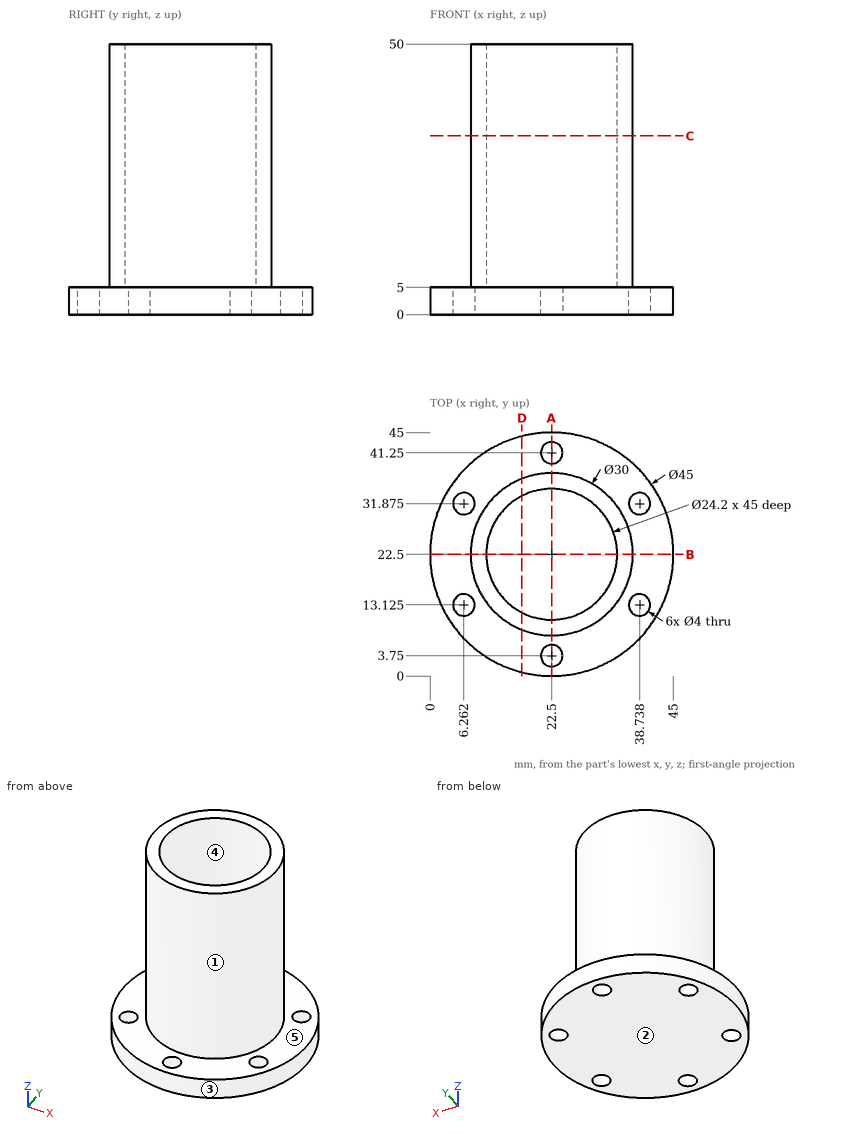
Design review of the part shown in the three views and the two pictorial views. Dimensions are in mm from the part's minimum x, y and z. A direction names the side the tool comes from. Round coordinates to 2 decimals unless told otherwise and drop trailing zeros. Write each loop counter-clockwise with the first axis right and the second up, starting at its lowest first coordinate (ties: lowest second). Pieces come first, ordered by that corner, then holes. Notation, with made-up numbers: (-38.5, 77) -> (6.5, 77) arc R23 ccw to (6.5, 95) -> close; hole circle Ø2 at (-7.5, -27.75). An arc over 180 degrees is marked (long way). Use one line per item in the form item = value.
1) Clearance check with flat-ended pins moving along their axes: pin 1 (4.5 mm diameter, centred on x = 22.5, y = 41.25, fed in from +Z); pin 2 (3 mm diameter, centred on x = 38.5, y = 16.5, fed in from -Z); pin 3 (3 mm diameter, centred on y = 16.5, z = 7, fed in from +X); pin 4 (4 mm diameter, centred on x = 12.5, z = 43.5, fed in from -Y). State where each tip first meets the part, or that it passes through.
Found:
pin_1 = 5
pin_2 = 0
pin_3 = 36.81
pin_4 = 9.81
2) Mouldability with a two-part tool opening along Y and no side actions: class the marked faces 3, 4 and 5 as +Y half, -Y half, draft (parallel to the pull), parting line (faces both ways), or undercut.
Found:
face_3 = parting line
face_4 = undercut
face_5 = draft
3) Tool access review of the marked faces 1 and 2: name each direction out of +Z, -Z, +X, -X, +Y, -Y from which nothing blocks a thin tool from reaching the whole face with its end or side.
Found:
face_1 = +Z
face_2 = -Z, +X, -X, +Y, -Y
4) Take a section at D-D, the plane x = 17. Write out the cut boundary in (y, z), and give its area (3 significant figures).
Found:
outline = (0.68, 0) -> (44.32, 0) -> (44.32, 5) -> (36.46, 5) -> (36.46, 50) -> (33.28, 50) -> (33.28, 5) -> (11.72, 5) -> (11.72, 50) -> (8.54, 50) -> (8.54, 5) -> (0.68, 5) -> close
area = 504 mm2
5) Take a section at C-C, the plane z = 33. Write out the cut boundary in (x, y).
Found:
outline = circle Ø30 at (22.5, 22.5); hole circle Ø24.2 at (22.5, 22.5)
6) To check wall thickness, follow L1, parallel to Y at x = 22.5, z = 1.4; L2, parallel to Y at x = 22, z = 25.5; L3, parallel to Z at x = 27.5, y = 16.5. State the ranges of each line that lie inside material, in increasing order. Write a range as from..to.
Found:
L1 = 0..1.75, 5.75..39.25, 43.25..45
L2 = 7.51..10.41, 34.59..37.49
L3 = 0..5
7) Take a section at A-A, the plane x = 22.5. Write out the cut boundary in (y, z), and give its area (3 significant figures).
Found:
outline = (0, 0) -> (1.75, 0) -> (1.75, 5) -> (0, 5) -> close; (5.75, 0) -> (39.25, 0) -> (39.25, 5) -> (37.5, 5) -> (37.5, 50) -> (34.6, 50) -> (34.6, 5) -> (10.4, 5) -> (10.4, 50) -> (7.5, 50) -> (7.5, 5) -> (5.75, 5) -> close; (43.25, 0) -> (45, 0) -> (45, 5) -> (43.25, 5) -> close
area = 446 mm2
8) Take a section at B-B, the plane y = 22.5. Write out the cut boundary in (x, z), and give its area (3 significant figures).
Found:
outline = (0, 0) -> (45, 0) -> (45, 5) -> (37.5, 5) -> (37.5, 50) -> (34.6, 50) -> (34.6, 5) -> (10.4, 5) -> (10.4, 50) -> (7.5, 50) -> (7.5, 5) -> (0, 5) -> close
area = 486 mm2
